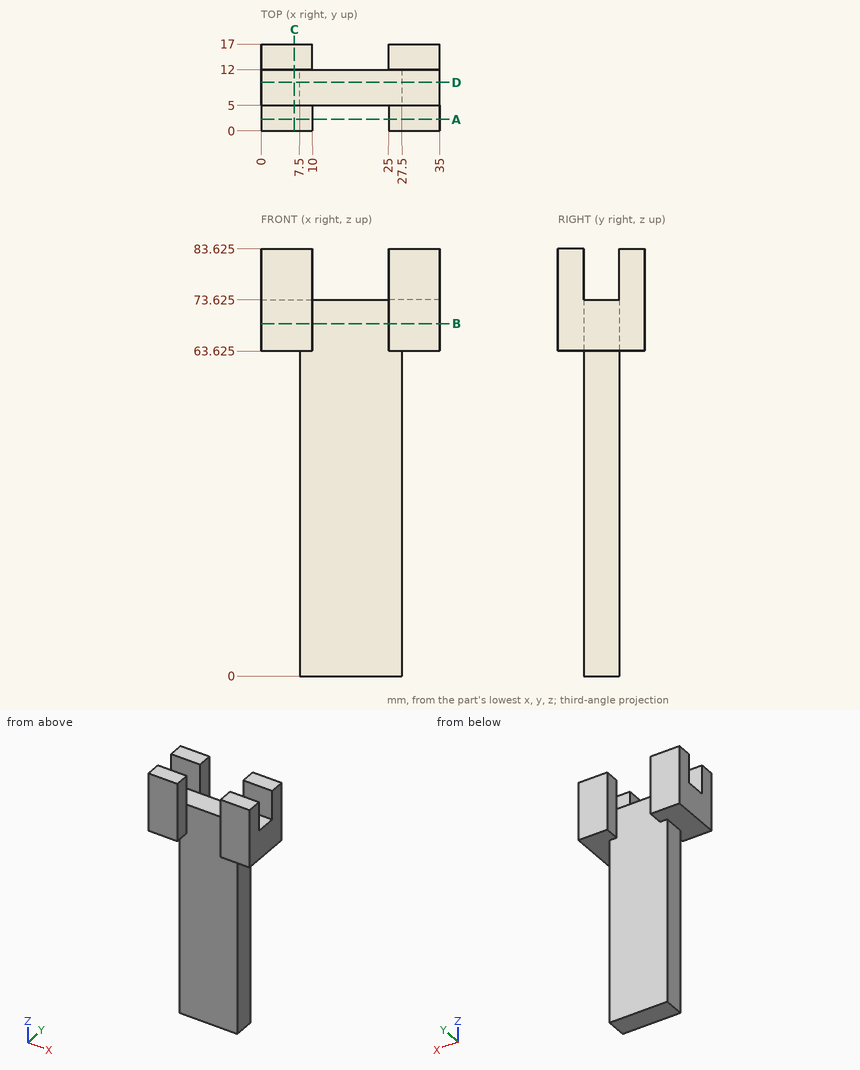
For this review, use the dimensioned drawing (mm, ordinates from the lowest corner) and the shaded views. Give positions to 0.01 mm unless a question says otherwise; leave off trailing zeros. Order: outer loops, then holes, each group sorted by start corner. A loop starts at its lowest first (then second) coordinate and runs counter-clockwise, first axis right, second up. Notation, with made-up numbers: M 23,-7 L 41,-7 A20 ccw 41,3 Z; hole C -25,42.25 d9. An arc over 180 degrees is marked long. One line per question, with ' | ' between items. Start each with the question number.
1) Consider section A-A, the plane y = 2.25. Give the boundary of the cut face in (x, z) (1 decimal).
2) Clearance check with flat-ended pins moving along their axes: P1, Ø3.5, axis at y = 8.5, z = 43.5, coming from the +X side; P2, Ø10, axis at x = 11.5, y = 7, coming from the -Z side; P3, Ø1.5, axis at x = 5, y = 10, coming from the -Z side (1 decimal); P4, Ø2, axis at x = 29, z = 43, coming from the -Y side. State where each tip first meets the part, or that it passes through.
3) Wall thickness on L1, parallel to X at y = 4.25, z = 74.5; L2, parallel to Z at x = 6.5, y = 10 (1 decimal); L3, parallel to Y at x = 19, z = 58.5: over which ranges is each line inside the solid? List them lowest first. Write a range as from..to.
4) Consider section B-B, the plane z = 69. Give the boundary of the cut face in (x, y), then the cut area to 3 significant figures.
5) Consider section D-D, the plane y = 9.5. Give the boundary of the cut face in (x, z) (1 decimal), then the cut area to 3 significant figures.
6) Consider section C-C, the plane x = 6.5. Give the boundary of the cut face in (y, z) (1 decimal), then the cut area to 3 significant figures.
Found:
1) outline: M 0,63.6 L 10,63.6 L 10,83.6 L 0,83.6 Z; M 25,63.6 L 35,63.6 L 35,83.6 L 25,83.6 Z
2) P1: stops at x = 27.5 | P2: stops at z = 0 | P3: stops at z = 63.6 | P4: passes through
3) L1: x = 0..10, 25..35 | L2: z = 63.6..73.6 | L3: y = 5..12
4) outline: M 0,0 L 10,0 L 10,5 L 25,5 L 25,0 L 35,0 L 35,17 L 25,17 L 25,12 L 10,12 L 10,17 L 0,17 Z | area: 445 mm²
5) outline: M 0,63.6 L 7.5,63.6 L 7.5,0 L 27.5,0 L 27.5,63.6 L 35,63.6 L 35,73.6 L 0,73.6 Z | area: 1,620 mm²
6) outline: M 0,63.6 L 17,63.6 L 17,83.6 L 12,83.6 L 12,73.6 L 5,73.6 L 5,83.6 L 0,83.6 Z | area: 270 mm²
